CAD build for the part. Positions are in the model's coordinates, mm. A direction names the side the tool comes from. Coordinates: 2 decimals unless noted, no trailing zeros. Loops run counter-clockwise (first coordinate to the right, second up) from the corner with the lowest first, then second, coordinate; pieces in that order, holes last.
1) Pin check, flat tips, straight feed: pin 1 Ø0.9 at (x, z) = (19, -2) entering from +Y; pin 2 Ø4 at (x, z) = (13, 144) entering from -Y; pin 3 Ø6 at (x, z) = (-8, 26) entering from +Y. Stop position of each tip, or through.
2) Which spindle directions (+Z, -Z, +X, -X, +Y, -Y) get a long thin tool onto all of the face, cutting with end or side? Do faces 1 (the flat face through (0, 0, 203)), 2 (the flat face through (5, 10, 190)). Say none if no direction does.
3) Two-plate mould, pull along Y, no slides. Class faces 3 (the cylindrical face through (0, -17, 94)), 4 (the flat face through (0, -8, -3)), 5 (the cylindrical face through (2.38, 10.74, 195.07)), 6 (the flat face through (0, 0, 200)): +Y half, -Y half, draft (parallel to the pull), parting line (faces both ways), or undercut.
4) Saw through at A-A, the plane x = 0. Write the cut outline in (y, z).
5) Saw through at B-B, the plane y = -6.5. Write the cut outline in (x, z).
6) Wall check: line 1 along Z through (x, y) = (-10, -6); line 2 along Z through (x, y) = (7, -6.5); line 3 along Y through (x, z) = (0, 195.5). Give the ranges that are in metal, low to high.
7) Saw through at D-D, the plane z = 27. Write the cut outline in (x, y).
8) Saw through at C-C, the plane y = 4. Write the cut outline in (x, z).
Autodesk Inventor part; units mm, degrees
ref_plane "YZ Plane" through (0, 0, 0) normal (1, 0, 0) x (0, 1, 0)
ref_plane "XZ Plane" through (0, 0, 0) normal (0, 1, 0) x (-1, 0, 0)
ref_plane "XY Plane" through (0, 0, 0) normal (0, 0, 1) x (1, 0, 0)
sketch "Sketch1" plane through (0, 0, 0) normal (0, 0, 1) x (1, 0, 0)
  arc A0 (-17, 0) -> (17, 0) centre (0, 0) ccw
  line L0 (-23.8, 0) -> (23.8, 0)
  line L1 (-17, 0) -> (17, 0)
  dimension "d1" = 17
extrude "Extrusion1" add sketch "Sketch1" along normal blind 200
shell "Shell1" thickness 3 outward yes removed faces 1 at (5.6667, 0, 66.6667)
sketch "Sketch2" plane through (0, 0, 200) normal (0, 0, -1) x (-1, 0, 0)
  circle A0 centre (0, 0) radius 20
  arc A1 (-20, 0) -> (20, 0) centre (0, 0) ccw
extrude "Extrusion2" add sketch "Sketch2" against normal up to surface (3 mm away)
sketch "Sketch3" plane through (0, 0, 200) normal (0, 0, -1) x (-1, 0, 0)
  circle A0 centre (0, 0) radius 11
  circle A1 centre (0, 0) radius 20
  circle A2 centre (0, 0) radius 20
  dimension "d7" = 22
extrude "Extrusion3" add sketch "Sketch3" along normal blind 10
properties part number "prototype3"
Data:
1. pin 1: stops at y = 0
1. pin 2: stops at y = -16.7
1. pin 3: stops at y = -12.96
2. face 1: +Z, +X, -X, +Y, -Y
2. face 2: +Y
3. face 3: +Y half
3. face 4: draft
3. face 5: undercut
3. face 6: undercut
4. outline: (-20, -3) - (0, -3) - (0, 0) - (-17, 0) - (-17, 190) - (-11, 190) - (-11, 200) - (11, 200) - (11, 190) - (20, 190) - (20, 203) - (-20, 203) - close
5. outline: (-18.91, -3) - (18.91, -3) - (18.91, 203) - (-18.91, 203) - close; hole (-15.71, 0) - (15.71, 0) - (15.71, 190) - (8.87, 190) - (8.87, 200) - (-8.87, 200) - (-8.87, 190) - (-15.71, 190) - close
6. line 1: z = -3 to 0, 190 to 203
6. line 2: z = -3 to 0, 200 to 203
6. line 3: y = -20 to -11, 11 to 20
7. outline: (-20, 0) arc R20 ccw to (20, 0) - (17, 0) arc R17 cw to (-17, 0) - close
8. outline: (-19.6, 190) - (-10.25, 190) - (-10.25, 200) - (10.25, 200) - (10.25, 190) - (19.6, 190) - (19.6, 203) - (-19.6, 203) - close
